from build123d import *

# Parameters (mm, degrees)
SKETCH1_R           = 30
BOSS_EXTRUDE1_DEPTH = 19
CUT_EXTRUDE1_START  = -2
SKETCH2_R           = 30
SKETCH2_R_2         = 25
CUT_EXTRUDE1_DEPTH  = 2
SKETCH3_R           = 30
SKETCH3_R_2         = 25
CUT_EXTRUDE2_DEPTH  = 2
CUT_EXTRUDE3_DEPTH  = 6.5
CUT_EXTRUDE4_REACH  = 48.487
SKETCH11_R          = 16
CUT_EXTRUDE5_REACH  = 48.487
SKETCH12_R          = 15
CUT_EXTRUDE6_START  = -2
SKETCH13_R          = 16
CUT_EXTRUDE6_DEPTH  = 2
SKETCH14_R          = 2
CUT_EXTRUDE7_DEPTH  = 3
CUT_EXTRUDE8_START  = -3
SKETCH15_R          = 1.5
SKETCH15_R_2        = 15
CUT_EXTRUDE8_DEPTH  = 3


with BuildPart() as part:
    # Sketch1 → Boss-Extrude1 (new body)
    with BuildSketch(Plane.XY):
        Circle(SKETCH1_R)
    extrude(amount=BOSS_EXTRUDE1_DEPTH)

    # Sketch2 → Cut-Extrude1 (cut)
    with BuildSketch(Plane.XY.offset(19).offset(CUT_EXTRUDE1_START)):
        Circle(SKETCH2_R)
        Circle(SKETCH2_R_2, mode=Mode.SUBTRACT)
    extrude(amount=CUT_EXTRUDE1_DEPTH, mode=Mode.SUBTRACT)

    # Sketch3 → Cut-Extrude2 (cut)
    with BuildSketch(Plane(origin=(0, 0, 0), x_dir=(-1, 0, 0), z_dir=(0, 0, -1))):
        Circle(SKETCH3_R)
        with Locations(Location((0, 0, 0), (0, 0, 180))):
            Circle(SKETCH3_R_2, mode=Mode.SUBTRACT)
    extrude(amount=-CUT_EXTRUDE2_DEPTH, mode=Mode.SUBTRACT)

    # Sketch10 → Cut-Extrude3 (cut, symmetric)
    with BuildSketch(Plane.XY.offset(9.5)):
        with BuildLine():
            Line((-7.071067812, -12.928932188), (-7.071067812, -29.154759474))
            ThreePointArc((-7.071067812, -29.154759474), (-28.265076636, 10.054125657), (12.928932188, 27.071067812))
            Line((12.928932188, 27.071067812), (7.071067812, 21.213203436))
            ThreePointArc((7.071067812, 21.213203436), (11.406522838, -0.582600835), (-7.071067812, -12.928932188))
        make_face()
    extrude(amount=CUT_EXTRUDE3_DEPTH, both=True, mode=Mode.SUBTRACT)

    # Sketch11 → Cut-Extrude4 (cut, up to next)
    with BuildSketch(Plane.XY.offset(19), mode=Mode.PRIVATE) as cut_extrude4_sk1:
        with Locations((-4.949747468, 4.949747468)):
            Circle(SKETCH11_R)
    cut_extrude4_tool1 = extrude(cut_extrude4_sk1.sketch, amount=-CUT_EXTRUDE4_REACH, mode=Mode.PRIVATE) & part.part
    add(cut_extrude4_tool1.solids().sort_by_distance((-4.949747, 4.949747, 19))[0], mode=Mode.SUBTRACT)

    # Sketch12 → Cut-Extrude5 (cut, up to next)
    with BuildSketch(Plane(origin=(0, 0, 0), x_dir=(-1, 0, 0), z_dir=(0, 0, -1)), mode=Mode.PRIVATE) as cut_extrude5_sk1:
        with Locations((4.949747468, 4.949747468)):
            Circle(SKETCH12_R)
    cut_extrude5_tool1 = extrude(cut_extrude5_sk1.sketch, amount=-CUT_EXTRUDE5_REACH, mode=Mode.PRIVATE) & part.part
    add(cut_extrude5_tool1.solids().sort_by_distance((-4.949747, 4.949747, 0))[0], mode=Mode.SUBTRACT)

    # Sketch13 → Cut-Extrude6 (cut)
    with BuildSketch(Plane(origin=(0, 0, 0), x_dir=(-1, 0, 0), z_dir=(0, 0, -1)).offset(CUT_EXTRUDE6_START)):
        with Locations(Location((4.949747468, 4.949747468, 0), (0, 0, 180))):
            Circle(SKETCH13_R)
    extrude(amount=CUT_EXTRUDE6_DEPTH, mode=Mode.SUBTRACT)

    # Sketch14 → Cut-Extrude7 (cut)
    with BuildSketch(Plane.XY.offset(19)):
        with Locations((0, -20)):
            Circle(SKETCH14_R)
    extrude(amount=-CUT_EXTRUDE7_DEPTH, mode=Mode.SUBTRACT)

    # Sketch15 → Cut-Extrude8 (cut)
    with BuildSketch(Plane.XY.offset(19).offset(CUT_EXTRUDE8_START)):
        with Locations((-4.949747468, -17.277677021)):
            Circle(SKETCH15_R)
        with Locations(Location((-4.949747468, 4.949747468, 0), (0, 0, 180))):
            Circle(SKETCH15_R_2)
        with Locations((17.277677021, 4.949747468)):
            Circle(SKETCH15_R)
    extrude(amount=CUT_EXTRUDE8_DEPTH, mode=Mode.SUBTRACT)


solid = part.part
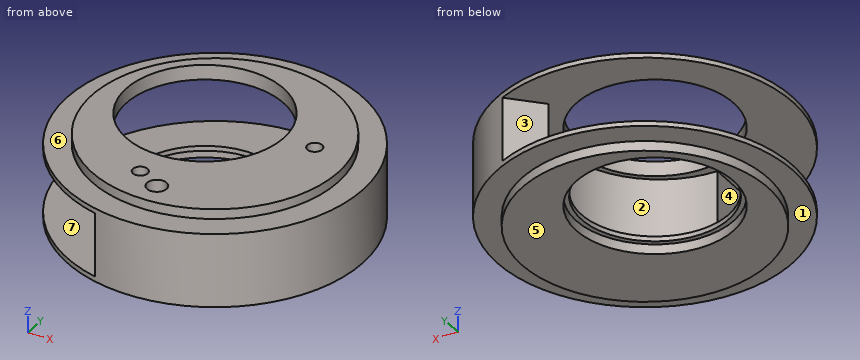
For this review, take the finished solid that the model builds, in its own axes (mm). Face numbers are marked on the shaded views. A direction names the side the tool comes from. Round coordinates to 2 decimals unless told otherwise and drop trailing zeros. Loops run counter-clockwise (first coordinate to the right, second up) from the corner with the lowest first, then second, coordinate; pieces in that order, holes last. Notation, with made-up numbers: (-7, 58.25) - (13, 58.25) arc R33 ccw to (13, 88.25) - close; hole circle Ø6 at (61.25, 79). An arc over 180 degrees is marked (long way). Answer as CSV lines item,"result".
(1) Consider section B-B on x = -12.5. Give the boundary of the cut face in (y, z).
Checked values:
outline,"(-27.27, 2) - (-21.65, 2) - (-21.65, 0) - (-9.16, 0) - (-9.16, 2) - (-8.01, 2) - (-8.01, 3) - (-27.27, 3) - close; (-27.27, 16) - (-9.16, 16) - (-9.16, 19) - (-21.65, 19) - (-21.65, 17) - (-27.27, 17) - close; (17.91, 2) - (19.06, 2) - (19.06, 0) - (21.65, 0) - (21.65, 2) - (27.27, 2) - (27.27, 3) - (17.91, 3) - close; (19.06, 16) - (27.27, 16) - (27.27, 17) - (21.65, 17) - (21.65, 19) - (19.06, 19) - close"
(2) Consider section C-C on x = 0. Give the number of separate pieces and of enclosed holes in the cut face, then the cut area to 3 significant figures.
Checked values:
separate pieces,"3"
enclosed holes,"0"
area,"366 mm2"
(3) Insertion check: P1, Ø1, axis at y = 20.5, z = 6, coming from the -X side; P2, Ø0.9, axis at x = -4.5, y = -17, coming from the +Z side; P3, Ø4, axis at y = 18, z = 9.5, coming from the -X side. Each pin has a flat end and moves straight along its axis. Give the tip position at first contact, or say it passes through.
Checked values:
P1,"stops at x = 7.28"
P2,"stops at z = 16"
P3,"stops at x = 8.19"
(4) Mouldability with a two-part tool opening along Z and no side actions: class the marked faces 4, 5, 6 and 7 as +Z half, -Z half, draft (parallel to the pull), parting line (faces both ways), or undercut.
Checked values:
face 4,"undercut"
face 5,"-Z half"
face 6,"+Z half"
face 7,"undercut"
(5) Wall thickness on line 1 (Z direction, x = -23.5, y = -2); line 2 (Z direction, x = -23.5, y = 11); line 3 (Z direction, x = 21, y = -18): over which ranges is each line inside the solid? List them lowest first.
Checked values:
line 1,"z = 0 to 3, 16 to 19"
line 2,"z = 2 to 3, 16 to 17"
line 3,"z = 2 to 17"
(6) Consider section D-D on z = 5.5. Give the boundary of the cut face in (x, y), then the cut area to 3 significant figures.
Checked values:
outline,"(-7.07, -29.15) arc R30 ccw to (12.93, 27.07) - (7.07, 21.21) arc R20 cw to (-7.07, -12.93) - close"
area,"1,120 mm2"
(7) Consider section A-A on y = 0. Give the boundary of the cut face in (x, z).
Checked values:
outline,"(-30, 2) - (-25, 2) - (-25, 0) - (-20.16, 0) - (-20.16, 2) - (-19.11, 2) - (-19.11, 3) - (-30, 3) - close; (-30, 16) - (-20.16, 16) - (-20.16, 19) - (-25, 19) - (-25, 17) - (-30, 17) - close; (9.21, 2) - (10.27, 2) - (10.27, 0) - (25, 0) - (25, 2) - (30, 2) - (30, 17) - (25, 17) - (25, 19) - (10.27, 19) - (10.27, 16) - (11.64, 16) - (11.64, 3) - (9.21, 3) - close"
(8) Tool access review of the marked faces 1, 2 and 3: name each direction out of +Z, -Z, +X, -X, +Y, -Y from which nothing blocks a thin tool from reaching the whole face with its end or side.
Checked values:
face 1,"-Z"
face 2,"-X"
face 3,"-X, +Y"
